```python
from build123d import *

# Parameters (mm, degrees)
SKETCH1_W                  = 86
SKETCH1_H                  = 68
BOSS_EXTRUDE1_DEPTH        = 6
SKETCH2_W                  = 10
SKETCH2_H                  = 25
SKETCH2_W_2                = 22
SKETCH2_H_2                = 15
CUT_EXTRUDE1_DEPTH         = 110.79981785
F_7_5_7_5_DIAMETER_HOLE1_D = 7.5
SKETCH234_W                = 10
SKETCH234_H                = 6
BOSS_EXTRUDE234_DEPTH      = 6
FILLET134_R                = 1
SKETCH2341_W               = 10
SKETCH2341_H               = 6
BOSS_EXTRUDE2341_DEPTH     = 6
FILLET1341_R               = 1
SKETCH2342_W               = 10
SKETCH2342_H               = 6
BOSS_EXTRUDE2342_DEPTH     = 6
FILLET1342_R               = 1
CUT_EXTRUDE11_START        = -3
SKETCH6_W                  = 10
SKETCH6_H                  = 6
CUT_EXTRUDE11_DEPTH        = 6
CUT_EXTRUDE16_DEPTH        = 82.966859266
CUT_EXTRUDE16_DEPTH_BACK   = 82.966859266
SKETCH64_W                 = 6
SKETCH64_H                 = 6
CUT_EXTRUDE18_DEPTH        = 101.225385192
CUT_EXTRUDE18_DEPTH_BACK   = 101.225385192
SKETCH66_W                 = 6
SKETCH66_H                 = 6
MIRROR2_OUTLINE_W          = 10
MIRROR2_OUTLINE_H          = 6
MIRROR2_OUTLINE_W_2        = 6
MIRROR2_DEPTH              = 6
MIRROR2_2_DEPTH            = 6


# Read off the part's stored shape, not the designer's step: Mirror2
with BuildPart() as part:
    # Sketch1 → Boss-Extrude1 (new body)
    with BuildSketch(Plane(origin=(0, 0, 0), x_dir=(1, 0, 0), z_dir=(0, 1, 0))):
        with Locations((43, -34)):
            Rectangle(SKETCH1_W, SKETCH1_H)
    extrude(amount=BOSS_EXTRUDE1_DEPTH)

    # Sketch2 → Cut-Extrude1 (cut, through all)
    with BuildSketch(Plane(origin=(0, 6, 0), x_dir=(1, 0, 0), z_dir=(0, 1, 0))):
        with Locations((19.6, -55.5)):
            Rectangle(SKETCH2_W, SKETCH2_H)
        with Locations((50.6, -60.5)):
            Rectangle(SKETCH2_W_2, SKETCH2_H_2)
    cut_extrude1 = extrude(amount=-CUT_EXTRUDE1_DEPTH, mode=Mode.SUBTRACT)

    # Mirror1: Cut-Extrude1 across plane
    add(cut_extrude1.mirror(Plane.XY.offset(34)), mode=Mode.SUBTRACT)

    # Ø7.5 (7.5) Diameter Hole1 (through all)
    with Locations(Plane(origin=(0, 0, 0), x_dir=(-1, 0, 0), z_dir=(0, -1, 0))):
        with Locations((-71, -34)):
            Hole(F_7_5_7_5_DIAMETER_HOLE1_D / 2)

    # Sketch234 → Boss-Extrude234 (add)
    with BuildSketch(Plane(origin=(73.032221392, 0, 68), x_dir=(1, 0, 0), z_dir=(0, 0, 1))):
        with Locations((0.767778608, 3)):
            Rectangle(SKETCH234_W, SKETCH234_H)
    extrude(amount=BOSS_EXTRUDE234_DEPTH)

    # Fillet134
    fillet134_edges = [part.edges().sort_by_distance(p)[0] for p in [
        (78.8, 3, 74),
        (68.8, 3, 74),
    ]]
    fillet(fillet134_edges, radius=FILLET134_R)

    # Sketch2341 → Boss-Extrude2341 (add)
    with BuildSketch(Plane(origin=(31.332221392, 0, 68), x_dir=(1, 0, 0), z_dir=(0, 0, 1))):
        with Locations((0.767778608, 3)):
            Rectangle(SKETCH2341_W, SKETCH2341_H)
    extrude(amount=BOSS_EXTRUDE2341_DEPTH)

    # Fillet1341
    fillet1341_edges = [part.edges().sort_by_distance(p)[0] for p in [
        (37.1, 3, 74),
        (27.1, 3, 74),
    ]]
    fillet(fillet1341_edges, radius=FILLET1341_R)

    # Sketch2342 → Boss-Extrude2342 (add)
    with BuildSketch(Plane(origin=(6.532221392, 0, 68), x_dir=(1, 0, 0), z_dir=(0, 0, 1))):
        with Locations((0.767778608, 3)):
            Rectangle(SKETCH2342_W, SKETCH2342_H)
    extrude(amount=BOSS_EXTRUDE2342_DEPTH)

    # Fillet1342
    fillet1342_edges = [part.edges().sort_by_distance(p)[0] for p in [
        (12.3, 3, 74),
        (2.3, 3, 74),
    ]]
    fillet(fillet1342_edges, radius=FILLET1342_R)

    # Sketch6 → Cut-Extrude11 (cut)
    with BuildSketch(Plane(origin=(73.032221392, 3, 13), x_dir=(1, 0, 0), z_dir=(0, 1, 0)).offset(CUT_EXTRUDE11_START)):
        with Locations((0.767778608, -44)):
            Rectangle(SKETCH6_W, SKETCH6_H)
    extrude(amount=CUT_EXTRUDE11_DEPTH, mode=Mode.SUBTRACT)

    # Sketch64 → Cut-Extrude16 (cut, two sides: drawn at the far end of the back side and taken through both)
    with BuildSketch(Plane(origin=(31.332221392, 3, 13), x_dir=(1, 0, 0), z_dir=(0, 1, 0)).offset(-CUT_EXTRUDE16_DEPTH_BACK)):
        with Locations((0.767778608, -44)):
            Rectangle(SKETCH64_W, SKETCH64_H)
    extrude(amount=CUT_EXTRUDE16_DEPTH + CUT_EXTRUDE16_DEPTH_BACK, mode=Mode.SUBTRACT)

    # Sketch66 → Cut-Extrude18 (cut, two sides: drawn at the far end of the back side and taken through both)
    with BuildSketch(Plane(origin=(6.532221392, 3, 13), x_dir=(1, 0, 0), z_dir=(0, 1, 0)).offset(-CUT_EXTRUDE18_DEPTH_BACK)):
        with Locations((0.767778608, -44)):
            Rectangle(SKETCH66_W, SKETCH66_H)
    extrude(amount=CUT_EXTRUDE18_DEPTH + CUT_EXTRUDE18_DEPTH_BACK, mode=Mode.SUBTRACT)

    # Mirror2 outline → Mirror2 (cut)
    with BuildSketch(Plane(origin=(0, 0, 0), x_dir=(1, 0, 0), z_dir=(0, 1, 0))):
        with Locations((73.8, -11)):
            Rectangle(MIRROR2_OUTLINE_W, MIRROR2_OUTLINE_H)
        with Locations((32.1, -11)):
            Rectangle(MIRROR2_OUTLINE_W_2, MIRROR2_OUTLINE_H)
        with Locations((7.3, -11)):
            Rectangle(MIRROR2_OUTLINE_W_2, MIRROR2_OUTLINE_H)
    extrude(amount=MIRROR2_DEPTH, mode=Mode.SUBTRACT)

    # Mirror2 2 outline → Mirror2 2 (add)
    with BuildSketch(Plane(origin=(0, 0, 0), x_dir=(1, 0, 0), z_dir=(0, 1, 0))):
        with BuildLine():
            Line((68.8, 0), (78.8, 0))
            Line((78.8, 0), (78.8, 5))
            ThreePointArc((78.8, 5), (78.507106781, 5.707106781), (77.8, 6))
            Line((77.8, 6), (69.8, 6))
            ThreePointArc((69.8, 6), (69.092893219, 5.707106781), (68.8, 5))
            Line((68.8, 5), (68.8, 0))
        make_face()
        with BuildLine():
            Line((27.1, 0), (37.1, 0))
            Line((37.1, 0), (37.1, 5))
            ThreePointArc((37.1, 5), (36.807106781, 5.707106781), (36.1, 6))
            Line((36.1, 6), (28.1, 6))
            ThreePointArc((28.1, 6), (27.392893219, 5.707106781), (27.1, 5))
            Line((27.1, 5), (27.1, 0))
        make_face()
        with BuildLine():
            Line((2.3, 0), (12.3, 0))
            Line((12.3, 0), (12.3, 5))
            ThreePointArc((12.3, 5), (12.007106781, 5.707106781), (11.3, 6))
            Line((11.3, 6), (3.3, 6))
            ThreePointArc((3.3, 6), (2.592893219, 5.707106781), (2.3, 5))
            Line((2.3, 5), (2.3, 0))
        make_face()
    extrude(amount=MIRROR2_2_DEPTH)


solid = part.part
```
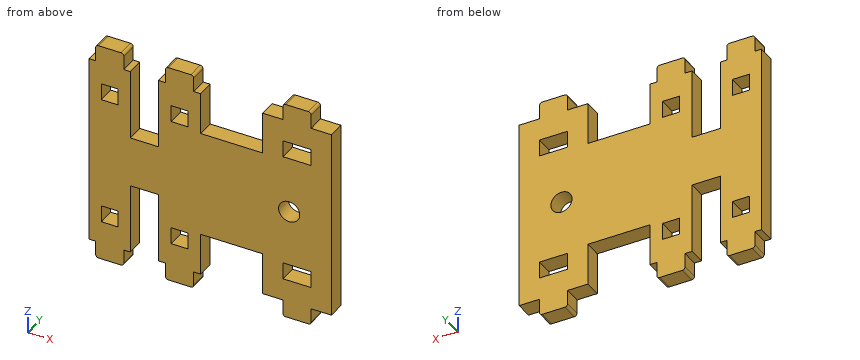
Read the model definition and answer for the solid it produces. Units are mm, in the model's axes. Coordinates: 2 decimals unless noted, no trailing zeros. Loops run counter-clockwise (first coordinate to the right, second up) from the corner with the lowest first, then second, coordinate; pieces in that order, holes last. Notation, with made-up numbers: (11.25, 10) - (15.25, 10) arc R28 cw to (15.25, 42) - close; hole circle Ø5 at (2.25, 27.5). An arc over 180 degrees is marked (long way). Answer in a Markdown table with one row per item.
1. Given pin 1 (1.2 mm diameter, centred on x = 1.5, y = 2.5, fed in from +Z); pin 2 (2.5 mm diameter, centred on y = 3.5, z = 70, fed in from +X); pin 3 (2.5 mm diameter, centred on y = 4, z = -3.5, fed in from -X), each flat-ended and moving along its own axis, determine where each tip first touches the part or whether it passes through.
Conclusion:
| item | result |
|---|---|
| pin 1 | stops at z = 68 |
| pin 2 | stops at x = 78.8 |
| pin 3 | stops at x = 2.3 |
2. Find section B-B, the plane x = 7.5. Write down the section's boundary in (y, z).
Conclusion:
| item | result |
|---|---|
| outline | (0, -6) - (6, -6) - (6, 8) - (0, 8) - close; (0, 14) - (6, 14) - (6, 54) - (0, 54) - close; (0, 60) - (6, 60) - (6, 74) - (0, 74) - close |
3. Find section D-D, the plane z = 34. Write down the section's boundary in (x, y).
Conclusion:
| item | result |
|---|---|
| outline | (0, 0) - (67.25, 0) - (67.25, 6) - (0, 6) - close; (74.75, 0) - (86, 0) - (86, 6) - (74.75, 6) - close |
4. Straight lines are drawn through the part: line 1 (X direction, y = 2.6, z = 67); line 2 (X direction, y = 5.65, z = 70); line 3 (Z direction, x = 71, y = 3.85). For each, find the intervals that lie inside material, in ascending order.
Conclusion:
| item | result |
|---|---|
| line 1 | x = 0 to 14.6, 24.6 to 39.6, 61.6 to 86 |
| line 2 | x = 2.3 to 12.3, 27.1 to 37.1, 68.8 to 78.8 |
| line 3 | z = -6 to 8, 14 to 30.25, 37.75 to 54, 60 to 74 |
5. Find section A-A, the plane x = 71. Write down the section's boundary in (y, z).
Conclusion:
| item | result |
|---|---|
| outline | (0, -6) - (6, -6) - (6, 8) - (0, 8) - close; (0, 14) - (6, 14) - (6, 30.25) - (0, 30.25) - close; (0, 37.75) - (6, 37.75) - (6, 54) - (0, 54) - close; (0, 60) - (6, 60) - (6, 74) - (0, 74) - close |
6. Find section C-C, the plane z = 16.5. Write down the section's boundary in (x, y), then the cut area to 3 significant figures.
Conclusion:
| item | result |
|---|---|
| outline | (0, 0) - (14.6, 0) - (14.6, 6) - (0, 6) - close; (24.6, 0) - (86, 0) - (86, 6) - (24.6, 6) - close |
| area | 456 mm² |
